The listing builds one solid part. Answer for the finished solid, in the listing's coordinates (mm). Give positions to 0.01 mm unless a question says otherwise; leave off trailing zeros. Loops run counter-clockwise (first coordinate to the right, second up) from the corner with the lowest first, then second, coordinate; pieces in that order, holes last. Notation, with made-up numbers: M 44,-12.75 L 55,-12.75 A32 cw 55,25.25 Z; hole C 3,-6 d4. An arc over 180 degrees is marked long. Return JSON: item names as keys, results as strings.
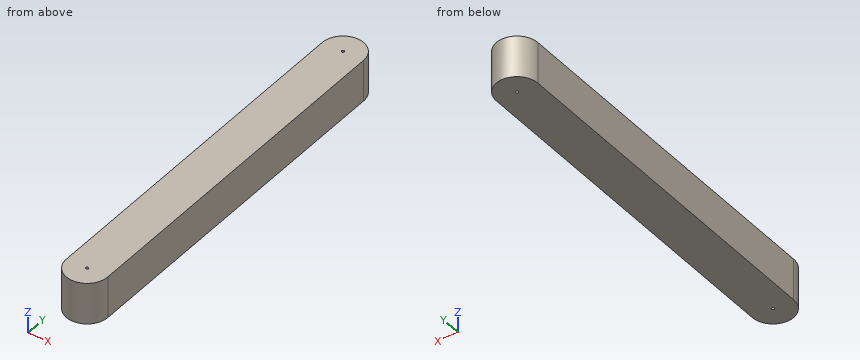
Autodesk Inventor part; units mm, degrees
ref_plane "YZ Plane" through (0, 0, 0) normal (1, 0, 0) x (0, 1, 0)
ref_plane "XZ Plane" through (0, 0, 0) normal (0, 1, 0) x (-1, 0, 0)
ref_plane "XY Plane" through (0, 0, 0) normal (0, 0, 1) x (1, 0, 0)
sketch "Sketch1" plane through (0, 0, 0) normal (0, 0, 1) x (1, 0, 0)
  circle A0 centre (0, -75) radius 5
  arc A1 (-75, -75) -> (75, -75) centre (0, -75) ccw
  line L0 (-75, -75) -> (-75, 1225)
  arc A2 (75, 1225) -> (-75, 1225) centre (0, 1225) ccw
  circle A3 centre (0, 1225) radius 5
  line L1 (75, 1225) -> (75, -75)
  point P0 (0, 0)
  dimension "d0" = 10
  dimension "d1" = 150
  dimension "d3" = 1300
  dimension "d4" = 75
extrude "Extrusion1" add sketch "Sketch1" along normal blind 150
properties part number "link2"
(1) Straight lines are drawn through the part: line 1 along Y through (x, z) = (0, 84); line 2 along X through (y, z) = (1225, 100); line 3 along Y through (x, z) = (-68, 125.5). For each, find the intervals that lie inside material, in ascending order.
Values follow:
{"line 1": "-150 to -80, -70 to 1220, 1230 to 1300", "line 2": "-75 to -5, 5 to 75", "line 3": "-106.64 to 1256.64"}
(2) The part is cut by section B-B (x = -42). Determine the outline of the cut face in (y, z).
Values follow:
{"outline": "M -137.14,0 L 1287.14,0 L 1287.14,150 L -137.14,150 Z"}
(3) Given pin 1 (10 mm diameter, centred on x = 53, z = 73, fed in from -Y), flat-ended and moving along its own axis, determine where the tip first touches the part or whether it passes through.
Values follow:
{"pin 1": "y = -132.63"}
(4) The part is cut by section A-A (z = 29). Determine the outline of the cut face in (x, y).
Values follow:
{"outline": "M -75,-75 A75 ccw 75,-75 L 75,1225 A75 ccw -75,1225 Z; hole C 0,-75 d10; hole C 0,1225 d10"}
